Could you check a few things on this model? Use its own coordinates, in mm. A direction names the side the tool comes from. Give positions to 0.01 mm unless a question says otherwise; leave off trailing zeros. Order: outer loops, then holes, each group sorted by start corner. A loop starts at its lowest first (then second) coordinate and runs counter-clockwise, first axis right, second up. Notation, with made-up numbers: (28.25, 8.25) -> (62.25, 8.25) arc R16 ccw to (62.25, 35.25) -> close; hole circle Ø5 at (62, -18.5). An arc over 180 degrees is marked (long way). One line per item, written item: value.
```python
from build123d import *

# Parameters (mm, degrees)
BOSS_EXTRUDE1_DEPTH = 23.38
SKETCH2_R           = 0.5
CUT_EXTRUDE1_DEPTH  = 44.5
SKETCH3_R           = 1
SKETCH3_R_2         = 3.935
CUT_EXTRUDE2_DEPTH  = 20.5


with BuildPart() as part:
    # Sketch1 → Boss-Extrude1 (new body)
    with BuildSketch(Plane.XY):
        Polygon((0, 0), (-14.37, 0), (-14.37, 9.76), (-12.75, 9.76), (-12.75, 1.62), (0, 1.62), align=None)
    boss_extrude1 = extrude(amount=BOSS_EXTRUDE1_DEPTH)

    # Sketch2 → Cut-Extrude1 (cut)
    with BuildSketch(Plane.ZY.offset(14.37)):
        with Locations((1.715, 5.81)):
            Circle(SKETCH2_R)
        with Locations((21.665, 5.81)):
            Circle(SKETCH2_R)
        with BuildLine():
            Line((6.539942279, 7.163555861), (16.840057721, 7.163555861))
            ThreePointArc((16.840057721, 7.163555861), (19.861748759, 9.087147646), (23.38, 9.76))
            Line((23.38, 9.76), (23.38, 14.744822673))
            Line((23.38, 14.744822673), (0, 14.744822673))
            Line((0, 14.744822673), (0, 9.76))
            ThreePointArc((0, 9.76), (3.518251241, 9.087147646), (6.539942279, 7.163555861))
        make_face()
    cut_extrude1 = extrude(amount=-CUT_EXTRUDE1_DEPTH, mode=Mode.SUBTRACT)

    # Mirror1: Boss-Extrude1, Cut-Extrude1 across plane
    add(boss_extrude1.mirror(Plane(origin=(0, 1.62, 23.38), x_dir=(0, 0, 1), z_dir=(-1, 0, 0))))
    add(cut_extrude1.mirror(Plane(origin=(0, 1.62, 23.38), x_dir=(0, 0, 1), z_dir=(-1, 0, 0))), mode=Mode.SUBTRACT)

    # Sketch3 → Cut-Extrude2 (cut)
    with BuildSketch(Plane(origin=(0, 0, 0), x_dir=(1, 0, 0), z_dir=(0, 1, 0))):
        with Locations((-7.071067812, -11.69)):
            Circle(SKETCH3_R)
        with Locations((7.071067812, -11.69)):
            Circle(SKETCH3_R)
        with Locations((5, -6.69)):
            Circle(SKETCH3_R)
        with Locations((-5, -6.69)):
            Circle(SKETCH3_R)
        with Locations((0, -11.69)):
            Circle(SKETCH3_R_2)
        with Locations((-5, -16.69)):
            Circle(SKETCH3_R)
        with Locations((5, -16.69)):
            Circle(SKETCH3_R)
        with Locations((0, -18.761067812)):
            Circle(SKETCH3_R)
        with Locations((0, -4.618932188)):
            Circle(SKETCH3_R)
    extrude(amount=CUT_EXTRUDE2_DEPTH, mode=Mode.SUBTRACT)


solid = part.part
```
1) We'd pull the mould along Z, two halves only. Please class faces 1 (the cylindrical face through (13.571, 9.106, 3.471)), 2 (the cylindrical face through (0.46, 0.8, 19.65)), 3 (the flat face through (-12.75, 5, 12)), 4 (the flat face through (-2, 1, 23.38)): +Z half, -Z half, draft (parallel to the pull), parting line (faces both ways), or undercut.
Answer below:
face 1: undercut
face 2: undercut
face 3: draft
face 4: +Z half
2) For P1, Ø0.8, axis at x = -13.5, z = 12, coming from the +Y side; P2, Ø1.2, axis at x = 0, z = 18.76, coming from the +Y side; P3, Ø7, axis at x = -1, z = 9.5, coming from the +Y side, each with a flat end and sliding along its axis, tell me the tip position at first contact or that it passes through.
Answer below:
P1: stops at y = 7.16
P2: passes through
P3: stops at y = 1.62
3) Suppose I cut it at B-B, the plane x = 0. Write out the boundary of the cut face in (y, z) (3 decimals), then the cut area to 3 significant figures.
Answer below:
outline: (0, 0) -> (1.62, 0) -> (1.62, 3.619) -> (0, 3.619) -> close; (0, 5.619) -> (1.62, 5.619) -> (1.62, 7.755) -> (0, 7.755) -> close; (0, 15.625) -> (1.62, 15.625) -> (1.62, 17.761) -> (0, 17.761) -> close; (0, 19.761) -> (1.62, 19.761) -> (1.62, 23.38) -> (0, 23.38) -> close
area: 18.6 mm2
4) Suppose I cut it at A-A, the plane y = 2.25. Write out the boundary of the cut face in (x, z), then the cut area to 3 significant figures.
Answer below:
outline: (-14.37, 0) -> (-12.75, 0) -> (-12.75, 23.38) -> (-14.37, 23.38) -> close; (12.75, 0) -> (14.37, 0) -> (14.37, 23.38) -> (12.75, 23.38) -> close
area: 75.8 mm2
5) For faces 5 (the cylindrical face through (-13.571, 5.832, 1.215)), 6 (the cylindrical face through (13.571, 9.068, 19.815)), which set-ups out of +Z, -Z, +X, -X, +Y, -Y let a thin tool reach every point of the face, with its end or its side?
Answer below:
face 5: +X, -X
face 6: +X, -X, +Y
6) Suppose I cut it at D-D, the plane z = 6. Write out the boundary of the cut face in (x, y), then the cut area to 3 significant figures.
Answer below:
outline: (-14.37, 0) -> (-5.72, 0) -> (-5.72, 1.62) -> (-12.75, 1.62) -> (-12.75, 7.64) -> (-14.37, 7.64) -> close; (-4.28, 0) -> (4.28, 0) -> (4.28, 1.62) -> (-4.28, 1.62) -> close; (5.72, 0) -> (14.37, 0) -> (14.37, 7.64) -> (12.75, 7.64) -> (12.75, 1.62) -> (5.72, 1.62) -> close
area: 61.4 mm2
7) Suppose I cut it at C-C, the plane y = 5.81. Write out the boundary of the cut face in (x, z) (3 decimals).
Answer below:
outline: (-14.37, 0) -> (-12.75, 0) -> (-12.75, 1.215) -> (-14.37, 1.215) -> close; (-14.37, 2.215) -> (-12.75, 2.215) -> (-12.75, 21.165) -> (-14.37, 21.165) -> close; (-14.37, 22.165) -> (-12.75, 22.165) -> (-12.75, 23.38) -> (-14.37, 23.38) -> close; (12.75, 0) -> (14.37, 0) -> (14.37, 1.215) -> (12.75, 1.215) -> close; (12.75, 2.215) -> (14.37, 2.215) -> (14.37, 21.165) -> (12.75, 21.165) -> close; (12.75, 22.165) -> (14.37, 22.165) -> (14.37, 23.38) -> (12.75, 23.38) -> close
8) If I drill on line 1 along X through (y, z) = (0.4, 11.69) (3 decimals); line 2 along Z through (x, y) = (-5, 0.65); line 3 along Z through (x, y) = (0, 0.65) (3 decimals), over which ranges is the centre line in solid material (lowest first)?
Answer below:
line 1: x = -14.37 to -8.071, -6.071 to -3.935, 3.935 to 6.071, 8.071 to 14.37
line 2: z = 0 to 5.69, 7.69 to 15.69, 17.69 to 23.38
line 3: z = 0 to 3.619, 5.619 to 7.755, 15.625 to 17.761, 19.761 to 23.38
